Verification items for the finished model (mm, model axes). A direction names the side the tool comes from. Give positions to 0.01 mm unless a question says otherwise; leave off trailing zeros. Order: outer loops, then holes, each group sorted by start corner. A loop starts at its lowest first (then second) coordinate and runs counter-clockwise, first axis right, second up. Notation, with made-up numbers: M 68.5,8.5 L 117.5,8.5 A15 ccw 117.5,27.5 Z; hole C -1.75,1 d1. An arc over 180 degrees is marked long. Answer as a JSON object with one key per item and string values.
```python
from build123d import *

# Parameters (mm, degrees)
SKETCH19_W               = 1030
SKETCH19_H               = 180
SKETCH19_W_2             = 1000
SKETCH19_H_2             = 150
BOSS_EXTRUDE2_DEPTH      = 48
SKETCH22_W               = 1030
SKETCH22_H               = 180
BOSS_EXTRUDE3_DEPTH      = 10
BOSS_EXTRUDE4_DEPTH      = 56
BOSS_EXTRUDE4_DEPTH_BACK = 10
SKETCH23_W               = 1500
SKETCH23_H               = 500
SKETCH23_W_2             = 1030
SKETCH23_H_2             = 180
CUT_EXTRUDE6_START       = 48
SKETCH26_R               = 1.65
CUT_EXTRUDE6_DEPTH       = 20
LPATTERN1_COUNT          = 5
LPATTERN1_PITCH          = 253.75
SKETCH28_R               = 2.3
SKETCH28_R_2             = 57.7
CUT_EXTRUDE7_DEPTH       = 793.55031386
LPATTERN2_COUNT          = 2
LPATTERN2_PITCH          = 350
LPATTERN2_COL_COUNT      = 2
LPATTERN2_COL_PITCH      = 350
CUT_EXTRUDE8_START       = 48
SKETCH27_R               = 1.65
CUT_EXTRUDE8_DEPTH       = 20
CUT_EXTRUDE9_START       = -56
CUT_EXTRUDE9_DEPTH       = 2
CUT_EXTRUDE10_START      = 56
CUT_EXTRUDE10_DEPTH      = 2
CUT_EXTRUDE11_DEPTH      = 793.55031386
CUT_EXTRUDE11_DEPTH_BACK = 793.55031386
SKETCH33_R               = 2.35
CUT_EXTRUDE12_DEPTH      = 793.55031386
CUT_EXTRUDE12_DEPTH_BACK = 793.55031386
SKETCH34_W               = 190.830831748
SKETCH34_H               = 540.530008981
SKETCH29_W               = 150
SKETCH29_H               = 100
BOSS_EXTRUDE5_DEPTH      = 50


with BuildPart() as part:
    # Sketch19 → Boss-Extrude2 (new body)
    with BuildSketch(Plane(origin=(0, 0, 0), x_dir=(1, 0, 0), z_dir=(0, 1, 0))):
        Rectangle(SKETCH19_W, SKETCH19_H)
        Rectangle(SKETCH19_W_2, SKETCH19_H_2, mode=Mode.SUBTRACT)
    extrude(amount=BOSS_EXTRUDE2_DEPTH)

    # Sketch22 → Boss-Extrude3 (add)
    with BuildSketch(Plane(origin=(0, 0, 0), x_dir=(1, 0, 0), z_dir=(0, 1, 0))):
        Rectangle(SKETCH22_W, SKETCH22_H)
    extrude(amount=-BOSS_EXTRUDE3_DEPTH)

    # Sketch23 → Boss-Extrude4 (add, two sides: drawn at the far end of the back side and taken through both)
    with BuildSketch(Plane(origin=(0, 0, 0), x_dir=(1, 0, 0), z_dir=(0, 1, 0)).offset(-BOSS_EXTRUDE4_DEPTH_BACK)):
        Rectangle(SKETCH23_W, SKETCH23_H)
        Rectangle(SKETCH23_W_2, SKETCH23_H_2, mode=Mode.SUBTRACT)
    extrude(amount=BOSS_EXTRUDE4_DEPTH + BOSS_EXTRUDE4_DEPTH_BACK)

    # Sketch26 → Cut-Extrude6 (cut)
    with BuildSketch(Plane(origin=(0, 0, 0), x_dir=(1, 0, 0), z_dir=(0, 1, 0)).offset(CUT_EXTRUDE6_START)):
        with Locations(Location((-507.5, -82.5, 0), (0, 0, 90))):
            Circle(SKETCH26_R)
        with Locations(Location((-507.5, 82.5, 0), (0, 0, 90))):
            Circle(SKETCH26_R)
    cut_extrude6 = extrude(amount=-CUT_EXTRUDE6_DEPTH, mode=Mode.SUBTRACT)

    # LPattern1: Cut-Extrude6 ×5
    with Locations(*[(i * LPATTERN1_PITCH, 0, 0) for i in range(1, LPATTERN1_COUNT)]):
        add(cut_extrude6, mode=Mode.SUBTRACT)

    # Sketch28 → Cut-Extrude7 (cut, symmetric)
    with BuildSketch(Plane(origin=(0, 0, 0), x_dir=(1, 0, 0), z_dir=(0, 1, 0))):
        with Locations(Location((-52.5, 52.5, 0), (0, 0, 270))):
            Circle(SKETCH28_R)
        with Locations(Location((52.5, 52.5, 0), (0, 0, 270))):
            Circle(SKETCH28_R)
        with Locations(Location((52.5, -52.5, 0), (0, 0, 270))):
            Circle(SKETCH28_R)
        with Locations(Location((-52.5, -52.5, 0), (0, 0, 270))):
            Circle(SKETCH28_R)
        with Locations(Location((0, 0, 0), (0, 0, 270))):
            Circle(SKETCH28_R_2)
    cut_extrude7 = extrude(amount=CUT_EXTRUDE7_DEPTH, both=True, mode=Mode.SUBTRACT)

    # LPattern2: Cut-Extrude7 ×2
    with Locations(*[(-i * LPATTERN2_PITCH, 0, 0) for i in range(1, LPATTERN2_COUNT)]):
        add(cut_extrude7, mode=Mode.SUBTRACT)

    # LPattern2 col: Cut-Extrude7 ×2
    with Locations(*[(i * LPATTERN2_COL_PITCH, 0, 0) for i in range(1, LPATTERN2_COL_COUNT)]):
        add(cut_extrude7, mode=Mode.SUBTRACT)

    # Sketch27 → Cut-Extrude8 (cut)
    with BuildSketch(Plane(origin=(0, 0, 0), x_dir=(1, 0, 0), z_dir=(0, 1, 0)).offset(CUT_EXTRUDE8_START)):
        with Locations(Location((-507.5, 27.5, 0), (0, 0, 90))):
            Circle(SKETCH27_R)
        with Locations(Location((-507.5, -35, 0), (0, 0, 90))):
            Circle(SKETCH27_R)
        with Locations(Location((507.5, -35, 0), (0, 0, 90))):
            Circle(SKETCH27_R)
        with Locations(Location((507.5, 27.5, 0), (0, 0, 90))):
            Circle(SKETCH27_R)
    extrude(amount=-CUT_EXTRUDE8_DEPTH, mode=Mode.SUBTRACT)

    # Sketch30 → Cut-Extrude9 (cut)
    with BuildSketch(Plane.XZ.offset(CUT_EXTRUDE9_START)):
        with BuildLine():
            Line((571.5, -147.92), (714.5, -147.92))
            ThreePointArc((714.5, -147.92), (715.207106781, -147.627106781), (715.5, -146.92))
            Line((715.5, -146.92), (715.5, -89.92))
            ThreePointArc((715.5, -89.92), (715.207106781, -89.212893219), (714.5, -88.92))
            Line((714.5, -88.92), (571.5, -88.92))
            ThreePointArc((571.5, -88.92), (567.964466094, -90.384466094), (566.5, -93.92))
            Line((566.5, -93.92), (566.5, -142.92))
            ThreePointArc((566.5, -142.92), (567.964466094, -146.455533906), (571.5, -147.92))
        make_face()
    cut_extrude9 = extrude(amount=CUT_EXTRUDE9_DEPTH, mode=Mode.SUBTRACT)

    # Mirror1: Cut-Extrude9 across plane
    add(cut_extrude9.mirror(Plane.XY), mode=Mode.SUBTRACT)

    # Sketch32 → Cut-Extrude10 (cut)
    with BuildSketch(Plane(origin=(0, 0, 0), x_dir=(1, 0, 0), z_dir=(0, 1, 0)).offset(CUT_EXTRUDE10_START)):
        with BuildLine():
            Line((-591.5, 147.92), (-571.5, 147.92))
            ThreePointArc((-571.5, 147.92), (-567.964466094, 146.455533906), (-566.5, 142.92))
            Line((-566.5, 142.92), (-566.5, 93.92))
            ThreePointArc((-566.5, 93.92), (-567.964466094, 90.384466094), (-571.5, 88.92))
            Line((-571.5, 88.92), (-591.5, 88.92))
            ThreePointArc((-591.5, 88.92), (-595.035533906, 90.384466094), (-596.5, 93.92))
            Line((-596.5, 93.92), (-596.5, 142.92))
            ThreePointArc((-596.5, 142.92), (-595.035533906, 146.455533906), (-591.5, 147.92))
        make_face()
    cut_extrude10 = extrude(amount=-CUT_EXTRUDE10_DEPTH, mode=Mode.SUBTRACT)

    # Mirror2: Cut-Extrude10 across plane
    add(cut_extrude10.mirror(Plane.XY), mode=Mode.SUBTRACT)

    # Sketch33 → Cut-Extrude11 (cut, two sides: drawn at the far end of the back side and taken through both)
    with BuildSketch(Plane(origin=(0, 0, 0), x_dir=(1, 0, 0), z_dir=(0, 1, 0)).offset(-CUT_EXTRUDE11_DEPTH_BACK)):
        with Locations(Location((-581.5, 108.58, 0), (0, 0, 270))):
            Circle(SKETCH33_R)
        with Locations(Location((-581.5, -108.59, 0), (0, 0, 270))):
            Circle(SKETCH33_R)
        with Locations(Location((-581.5, 128.25, 0), (0, 0, 270))):
            Circle(SKETCH33_R)
        with Locations(Location((-581.5, -128.26, 0), (0, 0, 270))):
            Circle(SKETCH33_R)
        with Locations(Location((616.17, -118.42, 0), (0, 0, 270))):
            Circle(SKETCH33_R)
        with Locations(Location((665.84, -118.42, 0), (0, 0, 270))):
            Circle(SKETCH33_R)
        with Locations(Location((616.17, 118.42, 0), (0, 0, 270))):
            Circle(SKETCH33_R)
        with Locations(Location((665.84, 118.42, 0), (0, 0, 270))):
            Circle(SKETCH33_R)
    extrude(amount=CUT_EXTRUDE11_DEPTH + CUT_EXTRUDE11_DEPTH_BACK, mode=Mode.SUBTRACT)

    # Sketch34 → Cut-Extrude12 (cut, two sides: drawn at the far end of the back side and taken through both)
    with BuildSketch(Plane(origin=(0, 0, 0), x_dir=(1, 0, 0), z_dir=(0, 1, 0)).offset(-CUT_EXTRUDE12_DEPTH_BACK)):
        with Locations((-726.415415874, 20.265004491)):
            Rectangle(SKETCH34_W, SKETCH34_H)
    extrude(amount=CUT_EXTRUDE12_DEPTH + CUT_EXTRUDE12_DEPTH_BACK, mode=Mode.SUBTRACT)

    # Sketch29 → Boss-Extrude5 (add)
    with BuildSketch(Plane(origin=(0, 0, 0), x_dir=(1, 0, 0), z_dir=(0, 1, 0))):
        with Locations((-556, -200)):
            Rectangle(SKETCH29_W, SKETCH29_H)
        with Locations((-556, 200)):
            Rectangle(SKETCH29_W, SKETCH29_H)
        with Locations((675, -200)):
            Rectangle(SKETCH29_W, SKETCH29_H)
        with Locations((675, 200)):
            Rectangle(SKETCH29_W, SKETCH29_H)
    extrude(amount=-BOSS_EXTRUDE5_DEPTH)


solid = part.part
```
Q1. Release check for a two-part mould opening along X. For faces 5 (the face through (-2, 48, -80)), 6 (the face through (750, 14, 3)), 7 (the face through (-631, 16, 3)), 8 (the face through (674, -50, -201)) record: +X half, -X half, draft (parallel to the pull), parting line (faces both ways), or undercut.
Resolved:
{"face 5": "undercut", "face 6": "+X half", "face 7": "-X half", "face 8": "draft"}
Q2. Section check C-C on y = -36.5. Record the cut outline in (x, z).
Resolved:
{"outline": "M -631,-250 L -481,-250 L -481,-150 L -631,-150 Z; M -631,150 L -481,150 L -481,250 L -631,250 Z; M 600,-250 L 750,-250 L 750,-150 L 600,-150 Z; M 600,150 L 750,150 L 750,250 L 600,250 Z"}
Q3. Section check B-B on z = 0. Record the cut outline in (x, y), then the cut area to 3 significant figures.
Resolved:
{"outline": "M -631,-10 L -407.7,-10 L -407.7,0 L -500,0 L -500,48 L -515,48 L -515,56 L -631,56 Z; M -292.3,-10 L -57.7,-10 L -57.7,0 L -292.3,0 Z; M 57.7,-10 L 292.3,-10 L 292.3,0 L 57.7,0 Z; M 407.7,-10 L 750,-10 L 750,56 L 515,56 L 515,48 L 500,48 L 500,0 L 407.7,0 Z", "area": "31,400 mm²"}
Q4. Gauge pin test, flat ends, axial feed: pin 1 Ø4 at (x, z) = (-183, 12.5) entering from -Y; pin 2 Ø8 at (x, z) = (95, -12) entering from +Y; pin 3 Ø2.5 at (x, z) = (-507.5, 82.5) entering from +Y. Record the tip position at first contact, or that the pin passes through.
Resolved:
{"pin 1": "stops at y = -10", "pin 2": "stops at y = 0", "pin 3": "stops at y = 28"}
Q5. Material ranges on L1, parallel to X at y = 15.5, z = -118.42; L2, parallel to Z at x = 0, y = 40.75; L3, parallel to X at y = 34, z = 35, recorded low to high.
Resolved:
{"L1": "x = -631 to 613.82, 618.52 to 663.49, 668.19 to 750", "L2": "z = -250 to -84.15, -80.85 to -75, 75 to 80.85, 84.15 to 250", "L3": "x = -631 to -509.15, -505.85 to -500, 500 to 505.85, 509.15 to 750"}
Q6. Tool access check on faces 1 (the face through (-557, -30, 150)), 2 (the face through (600, -30, 201)), 3 (the face through (50, 14, -250)), 4 (the face through (-581, 54, 119)). Record the directions out of +Z, -Z, +X, -X, +Y, -Y that give a thin tool (end or side, any length) a straight path to the whole face; none if there is none.
Resolved:
{"face 1": "+X, -X, -Y", "face 2": "+Z, -Z, -Y", "face 3": "-Z, +X, -X, +Y, -Y", "face 4": "+Y"}
Q7. Section check D-D on x = -123. Record the cut outline in (y, z).
Resolved:
{"outline": "M -10,-250 L 56,-250 L 56,-90 L 48,-90 L 48,-75 L 0,-75 L 0,75 L 48,75 L 48,90 L 56,90 L 56,250 L -10,250 Z"}
Q8. Section check A-A on x = -350. Record the cut outline in (y, z), then the cut area to 3 significant figures.
Resolved:
{"outline": "M -10,-250 L 56,-250 L 56,-90 L 48,-90 L 48,-75 L 0,-75 L 0,-57.7 L -10,-57.7 Z; M -10,57.7 L 0,57.7 L 0,75 L 48,75 L 48,90 L 56,90 L 56,250 L -10,250 Z", "area": "23,200 mm²"}
